from build123d import *

# Parameters (mm, degrees)
SKETCH_1_R               = 150
SKETCH_1_R_2             = 5
EXTRUDE_1_DEPTH          = 10
SKETCH_2_W               = 50
SKETCH_2_H               = 20
SKETCH_2_W_2             = 20
SKETCH_2_H_2             = 50
CUT_EXTRUDE_1_DEPTH      = 5
SKETCH_4_R               = 5
CUT_EXTRUDE_3_DEPTH      = 229.048761054
CUT_EXTRUDE_4_DEPTH      = 229.213140327
CUT_EXTRUDE_4_DEPTH_BACK = 229.213140327
SKETCH_3_W               = 20
SKETCH_3_H               = 50


with BuildPart() as part:
    # 草图1 → 凸台-拉伸1 (new body)
    with BuildSketch(Plane.XY):
        with Locations((-15.39076342, 6.930343762)):
            Circle(SKETCH_1_R)
        with Locations((-15.39076342, 6.930343762)):
            Circle(SKETCH_1_R_2, mode=Mode.SUBTRACT)
    extrude(amount=EXTRUDE_1_DEPTH)

    # 草图2 → 切除-拉伸1 (cut)
    with BuildSketch(Plane.XY.offset(10)):
        with Locations((99.60923658, 6.930343762)):
            Rectangle(SKETCH_2_W, SKETCH_2_H)
        with Locations((-15.39076342, 121.930343762)):
            Rectangle(SKETCH_2_W_2, SKETCH_2_H_2)
        with Locations((-15.39076342, -108.069656238)):
            Rectangle(SKETCH_2_W_2, SKETCH_2_H_2)
        with Locations((-130.39076342, 6.930343762)):
            Rectangle(SKETCH_2_W, SKETCH_2_H)
    extrude(amount=-CUT_EXTRUDE_1_DEPTH, mode=Mode.SUBTRACT)

    # 草图4 → 切除-拉伸3 (cut, through all)
    with BuildSketch(Plane.XY.offset(5)):
        with Locations((109.60923658, 6.930343762)):
            Circle(SKETCH_4_R)
        with Locations((-15.39076342, -118.069656238)):
            Circle(SKETCH_4_R)
        with Locations((-140.39076342, 6.930343762)):
            Circle(SKETCH_4_R)
        with Locations((-15.39076342, 131.930343762)):
            Circle(SKETCH_4_R)
    extrude(amount=-CUT_EXTRUDE_3_DEPTH, mode=Mode.SUBTRACT)

    # 草图3 → 切除-拉伸4 (cut, two sides: drawn at the far end of the back side and taken through both)
    with BuildSketch(Plane.XY.offset(10).offset(-CUT_EXTRUDE_4_DEPTH_BACK)):
        with Locations((44.60923658, 6.930343762)):
            Rectangle(SKETCH_3_W, SKETCH_3_H)
        with Locations((-75.39076342, 6.930343762)):
            Rectangle(SKETCH_3_W, SKETCH_3_H)
    extrude(amount=CUT_EXTRUDE_4_DEPTH + CUT_EXTRUDE_4_DEPTH_BACK, mode=Mode.SUBTRACT)


solid = part.part
Geometry: final body of the model. Coordinates: model frame, mm. A direction names the side the tool comes from. Round coordinates to 2 decimals unless told otherwise and drop trailing zeros. Loops run counter-clockwise (first coordinate to the right, second up) from the corner with the lowest first, then second, coordinate; pieces in that order, holes last.
Q1. Section B-B on z = 8. Return loops of the section in (x, y), plus the area to 3 significant figures.
Q2. Section D-D on x = 83. Return loops of the section in (y, z), plus the area to 3 significant figures.
Q3. Section A-A on x = -73. Return loops of the section in (y, z).
Q4. Access query for faces 4 (the flat face through (-76, -18.07, 5)), 5 (the flat face through (-16, -108, 5)), 6 (the flat face through (-17, -24, 10)). Directions: +Z, -Z, +X, -X, +Y, -Y. A direction counts if a zero-diameter tool reaches every point of the face in a straight line with its end or side. Return the directions, or none.
Q5. Section C-C on y = 116.5. Return loops of the section in (x, z), plus the area to 3 significant figures.
Q6. Material intervals for L1, parallel to X at y = -12.5, z = 4; L2, parallel to X at y = -1, z = 5.25; L3, parallel to Y at x = -21, z = 6.5, sorted ascending.
Q7. Pin query (flat end, axial travel): P1, Ø1.5, axis at x = -18.5, z = 7.5, coming from the -Y side; P2, Ø2.5, axis at y = 114, z = 6.5, coming from the +X side; P3, Ø11.5, axis at x = -140.39, y = 6.93, coming from the +Z side. Return the tip coordinate at first contact, or that it passes through.
Q8. Pull-direction query (Y, two-part tool) for faces 1 (the flat face through (-17, -24, 0)), 2 (the cylindrical face through (-47.908, -139.503, 4.93)), 3 (the flat face through (54.609, 7, 5)); classes: released by +Y, released by -Y, zero draft, split by the parting line, or undercut.
Evaluation:
1. outline: circle Ø300 at (-15.39, 6.93); hole (-155.39, -3.07) - (-105.39, -3.07) - (-105.39, 16.93) - (-155.39, 16.93) - close; hole (-85.39, -18.07) - (-65.39, -18.07) - (-65.39, 31.93) - (-85.39, 31.93) - close; hole (-25.39, -133.07) - (-5.39, -133.07) - (-5.39, -83.07) - (-25.39, -83.07) - close; hole (-25.39, 96.93) - (-5.39, 96.93) - (-5.39, 146.93) - (-25.39, 146.93) - close; hole circle Ø10 at (-15.39, 6.93); hole (34.61, -18.07) - (54.61, -18.07) - (54.61, 31.93) - (34.61, 31.93) - close; hole (74.61, -3.07) - (124.61, -3.07) - (124.61, 16.93) - (74.61, 16.93) - close
1. area: 64,600 mm2
2. outline: (-106.29, 0) - (120.15, 0) - (120.15, 10) - (16.93, 10) - (16.93, 5) - (-3.07, 5) - (-3.07, 10) - (-106.29, 10) - close
2. area: 2,160 mm2
3. outline: (-131.57, 0) - (-18.07, 0) - (-18.07, 10) - (-131.57, 10) - close; (31.93, 0) - (145.43, 0) - (145.43, 10) - (31.93, 10) - close
4. face 4: +Z, -Z
4. face 5: +Z
4. face 6: +Z, +X, -X, +Y, -Y
5. outline: (-117.83, 0) - (87.05, 0) - (87.05, 10) - (-5.39, 10) - (-5.39, 5) - (-25.39, 5) - (-25.39, 10) - (-117.83, 10) - close
5. area: 1,950 mm2
6. L1: x = -164.13 to -85.39, -65.39 to 34.61, 54.61 to 133.35
6. L2: x = -165.18 to -155.39, -105.39 to -85.39, -65.39 to 34.61, 54.61 to 74.61, 124.61 to 134.4
6. L3: y = -142.96 to -133.07, -83.07 to 96.93, 146.93 to 156.83
7. P1: stops at y = -143.05
7. P2: stops at x = 90.92
7. P3: stops at z = 5
8. face 1: zero draft
8. face 2: split by the parting line
8. face 3: undercut
